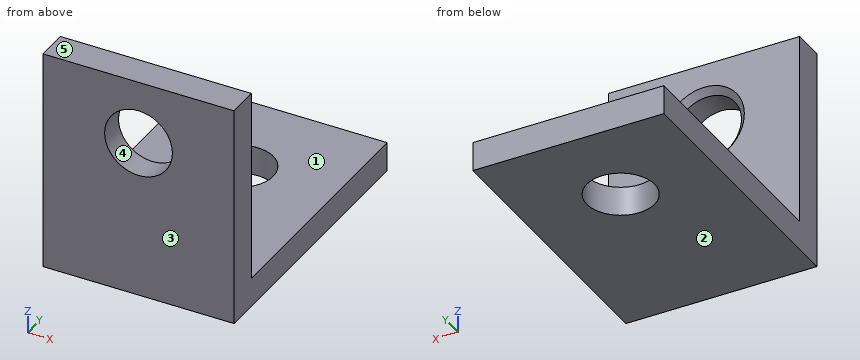
from build123d import *

# Parameters (mm, degrees)
SKETCH1_W               = 19.05
SKETCH1_H               = 22.225
BOSS_EXTRUDE1_DEPTH     = 3.175
SKETCH2_W               = 19.05
SKETCH2_H               = 3.175
BOSS_EXTRUDE2_DEPTH     = 24.765
F_1_4_CLEARANCE_HOLE3_D = 6.7564
MOVE_FACE1_BY           = 0.254


with BuildPart() as part:
    # Sketch1 → Boss-Extrude1 (new body)
    with BuildSketch(Plane(origin=(0, 0, 0), x_dir=(1, 0, 0), z_dir=(0, 1, 0))):
        with Locations((9.525, 11.1125)):
            Rectangle(SKETCH1_W, SKETCH1_H)
    extrude(amount=BOSS_EXTRUDE1_DEPTH)

    # Sketch2 → Boss-Extrude2 (add)
    with BuildSketch(Plane(origin=(0, 3.175, 0), x_dir=(1, 0, 0), z_dir=(0, 1, 0))):
        with Locations((9.525, 20.6375)):
            Rectangle(SKETCH2_W, SKETCH2_H)
    extrude(amount=BOSS_EXTRUDE2_DEPTH)

    # Sketch7 → 1/4 Clearance Hole2 (revolve, cut)
    with BuildSketch(Plane(origin=(9.525, 3.175, -6.35), x_dir=(0, 0, 1), z_dir=(1, 0, 0))):
        Polygon((0, 0), (0, 3.175), (3.3782, 3.175), (3.3782, 0.635), (4.0132, 0), align=None)
    revolve(axis=Axis((9.525, 9.525, -6.35), (0, -1, 0)), mode=Mode.SUBTRACT)

    # 1/4 Clearance Hole3 (through all)
    with Locations(Plane(origin=(9.525, 18.415, -19.05), x_dir=(1, 0, 0), z_dir=(0, 0, 1))):
        with Locations((0, 0)):
            Hole(F_1_4_CLEARANCE_HOLE3_D / 2)

    # Move Face1: a face moved inward by 0.254
    extrude(part.faces().sort_by_distance((9.525, 9.36625, -19.05))[0], amount=MOVE_FACE1_BY, dir=(0, 0, -1), mode=Mode.SUBTRACT)


solid = part.part
Part model, mm, in its own coordinate system. Face numbers are marked on the shaded views. A direction names the side the tool comes from. Coordinates: 2 decimals unless noted, no trailing zeros. Loops run counter-clockwise (first coordinate to the right, second up) from the corner with the lowest first, then second, coordinate; pieces in that order, holes last. Notation, with made-up numbers: (-0.5, -25.75) - (55.5, -25.75) arc R27 ccw to (55.5, 10.25) - close; hole circle Ø10 at (-14, 65.25). An arc over 180 degrees is marked (long way). Write each question's results on one line, items separated by ' | '. Start each with the question number.
Q1. Slice it at D-D on z = -18.75. Give the cut face in (x, y) (3 decimals).
Q2. Slice it at C-C on y = 14.25. Give the cut face in (x, z) (3 decimals), and give its area (3 significant figures).
Q3. Two-plate mould, pull along Z, no slides. Class the marked faces 3, 4 and 5: +Z half, -Z half, draft (parallel to the pull), parting line (faces both ways), or undercut.
Q4. Slice it at B-B on x = 3. Give the cut face in (y, z) (3 decimals), and give its area (3 significant figures).
Q5. Slice it at A-A on z = -6.35. Give the cut face in (x, y) (3 decimals).
Q6. Which spindle directions (+Z, -Z, +X, -X, +Y, -Y) get a long thin tool onto all of the face, cutting with end or side? Do the marked faces 1 and 2. Say none if no direction does.
Q7. Probe line 1 along X through (y, z) = (1.05, -6.35); line 2 along Z through (x, y) = (12.75, 12.25) (3 decimals); line 3 along Y through (x, z) = (18, -18.25) (3 decimals). List the from-to ranges inside material, lowest first.
Q8. Drop flat-ended pins along their axis: pin 1 Ø4 at (x, z) = (7, -13.5) entering from +Y (3 decimals); pin 2 Ø8 at (x, y) = (4, 19) entering from +Z. Give the stop position or say it passes through.
Answer:
1) outline: (0, 0) - (19.05, 0) - (19.05, 3.175) - (0, 3.175) - close
2) outline: (0, -22.225) - (19.05, -22.225) - (19.05, -19.304) - (0, -19.304) - close | area: 55.6 mm2
3) face 3: draft | face 4: undercut | face 5: +Z half
4) outline: (0, -22.225) - (27.94, -22.225) - (27.94, -19.304) - (3.175, -19.304) - (3.175, 0) - (0, 0) - close | area: 143 mm2
5) outline: (0, 0) - (6.147, 0) - (6.147, 2.54) - (5.512, 3.175) - (0, 3.175) - close; (12.903, 0) - (19.05, 0) - (19.05, 3.175) - (13.538, 3.175) - (12.903, 2.54) - close
6) face 1: +Z, +X, -X, +Y | face 2: -Z, +X, -X, +Y, -Y
7) line 1: x = 0 to 6.15, 12.9 to 19.05 | line 2: z = -22.225 to -19.304 | line 3: y = 0 to 3.175
8) pin 1: stops at y = 3.175 | pin 2: stops at z = -19.3
